Could you check a few things on this model? Use its own coordinates, in mm. A direction names the side the tool comes from. Give positions to 0.01 mm unless a question says otherwise; leave off trailing zeros. Loops run counter-clockwise (first coordinate to the right, second up) from the corner with the lowest first, then second, coordinate; pieces in that order, holes last. Notation, with made-up numbers: M 14,49 L 20,49 A9 ccw 20,57 Z; hole C 3.5,-30 d4. An arc over 180 degrees is marked long. Return JSON: item names as keys, results as strings. Group by question number.
1. For faces 4 (the flat face through (0, 5, 35)), 5 (the cylindrical face through (0.17, 9.82, -77.42)), 6 (the cylindrical face through (-1.183, 2.465, 90.145)), which set-ups out of +Z, -Z, +X, -X, +Y, -Y let a thin tool reach every point of the face, with its end or its side?
2. If we section it at A-A (z = 84): Write out the boundary of the cut face in (x, y), plus the area to 3 significant figures.
3. If we section it at D-D (z = -70.5): Write out the boundary of the cut face in (x, y), plus the area to 3 significant figures.
4. If we mould it in two halves opening along Z, with no side actions, what happens to faces 1 (the flat face through (0, 0, 21)), 2 (the cylindrical face through (0.168, 4.335, -77.402)), 3 (the cylindrical face through (-9.183, 2.465, 90.145))? For each: +Z half, -Z half, draft (parallel to the pull), parting line (faces both ways), or undercut.
5. If we section it at B-B (x = -8): Write out the boundary of the cut face in (y, z), plus the area to 3 significant figures.
6. If we section it at C-C (z = 49.5): Write out the boundary of the cut face in (x, y).
7. For pin 1 (2.5 mm diameter, centred on x = 0, z = 84, fed in from -Y); pin 2 (2.5 mm diameter, centred on x = 1, y = 8, fed in from +Z), each with a flat end and sliding along its axis, tell me the tip position at first contact or that it passes through.
8. Please list where these lines run through material, in increasing order: line 1 (Y direction, x = -4, z = 38); line 2 (Z direction, x = -3, y = 12.5); line 3 (Z direction, x = 10.75, y = 12).
Autodesk Inventor part; units mm, degrees
ref_plane "YZ Plane" through (0, 0, 0) normal (1, 0, 0) x (0, 1, 0)
ref_plane "XZ Plane" through (0, 0, 0) normal (0, 1, 0) x (-1, 0, 0)
ref_plane "XY Plane" through (0, 0, 0) normal (0, 0, 1) x (1, 0, 0)
sketch "Sketch1" plane through (0, 0, 0) normal (0, 1, 0) x (-1, 0, 0)
  line L0 (-10, 96) -> (10, 96)
  line L1 (12, 94) -> (12, -96)
  line L2 (12, -96) -> (-12, -96)
  line L3 (-12, -96) -> (-12, 94)
  line L4 (-12, 96) -> (12, -96) construction
  line L5 (12, 96) -> (-12, -96) construction
  arc A0 (12, 94) -> (10, 96) centre (10, 94) ccw
  arc A1 (-10, 96) -> (-12, 94) centre (-10, 94) ccw
  circle A2 centre (8, 92) radius 2.2
  circle A3 centre (0, 92) radius 2.2
  circle A4 centre (-8, 92) radius 2.2
  circle A5 centre (8, 84) radius 2.2
  circle A6 centre (0, 84) radius 2.2
  circle A7 centre (-8, 84) radius 2.2
  point P0 (0, 0)
  dimension "d0" = 24
  dimension "d1" = 192
  dimension "d2" = 2
  dimension "d3" = 4.4
  dimension "d4" = 4
  dimension "d5" = 4
  dimension "d8" = 8
  dimension "d11" = 8
extrude "Extrusion1" add sketch "Sketch1" along normal blind 5
sketch "Sketch2" plane through (12, 0, 94) normal (1, 0, 0) x (0, 0, -1)
  arc A0 (150, 5) -> (189.1089, 23.8473) centre (150, 55) ccw
  line L0 (0, 5) -> (190, 5)
  line L1 (190, 5) -> (190, 23.5357)
  arc A1 (190, 23.5357) -> (189.1089, 23.8473) centre (189.5, 23.5357) ccw
  point P0 (94, 0)
  point P1 (190, 25)
  dimension "d16" = 100
  dimension "d17" = 40
  dimension "d18" = 0.5
extrude "Extrusion2" add sketch "Sketch2" against normal blind 24
sketch "Sketch3" plane through (12, 0, 94) normal (1, 0, 0) x (0, 0, -1)
  line L0 (0, 0) -> (190, 0)
  arc A0 (150, 5) -> (189.1089, 23.8473) centre (150, 55) ccw
  line L1 (0, 5) -> (150, 5)
  arc A1 (150, 0) -> (189.8624, 17.1055) centre (150, 55) ccw
  line L2 (190, 0) -> (190, 23.5357)
  line L3 (190, 17.2508) -> (190, 0)
  line L4 (190, 0) -> (150, 0)
  arc A2 (189.8624, 17.1055) -> (190, 17.45) centre (189.5, 17.45) ccw
  point P0 (150, 0)
  dimension "d27" = 1
  dimension "d28" = 17.2508
extrude "Extrusion3" cut sketch "Sketch3" against normal blind 24
sketch "Sketch4" plane through (12, 0, 94) normal (1, 0, 0) x (0, 0, -1)
  arc A0 (122.7723, 13.0637) -> (150, 5) centre (150, 55) ccw
  line L0 (0, 5) -> (150, 5)
  line L1 (190, 17.45) -> (190, 23.5357)
  line L2 (122, 5) -> (122, 12.6444)
  arc A1 (122.7723, 13.0637) -> (122, 12.6444) centre (122.5, 12.6444) ccw
  point P0 (94, 0)
  point P1 (122, 13.5754)
  dimension "d31" = 0.5
extrude "Extrusion4" add sketch "Sketch4" against normal blind 24
properties part number "Launcher_Arm_V1"
Answer:
{
 "1": {"face 4": "+Z, +X, -X, +Y", "face 5": "+X, -X, +Y", "face 6": "+Y, -Y"},
 "2": {"outline": "M -12,0 L -10.2,0 L -10.2,5 L -12,5 Z; M -5.8,0 L -2.2,0 L -2.2,5 L -5.8,5 Z; M 2.2,0 L 5.8,0 L 5.8,5 L 2.2,5 Z; M 10.2,0 L 12,0 L 12,5 L 10.2,5 Z", "area": "54.0 mm²"},
 "3": {"outline": "M -12,1.95 L 12,1.95 L 12,7.15 L -12,7.15 Z", "area": "125 mm²"},
 "4": {"face 1": "draft", "face 2": "-Z half", "face 3": "undercut"},
 "5": {"outline": "M 0,-56 A55 ccw 17.11,-95.86 A0.5 ccw 17.45,-96 L 23.54,-96 A0.5 ccw 23.85,-95.11 A50 cw 5,-56 A50 cw 13.06,-28.77 A0.5 ccw 12.64,-28 L 5,-28 L 5,81.8 L 0,81.8 Z; M 0,86.2 L 5,86.2 L 5,89.8 L 0,89.8 Z; M 0,94.2 L 5,94.2 L 5,96 L 0,96 Z", "area": "1,020 mm²"},
 "6": {"outline": "M -12,0 L 12,0 L 12,5 L -12,5 Z"},
 "7": {"pin 1": "passes through", "pin 2": "stops at z = -28"},
 "8": {"line 1": "y = 0 to 5", "line 2": "z = -90.91 to -82.34, -29.66 to -28", "line 3": "z = -90.29 to -81.51, -30.49 to -28"}
}
